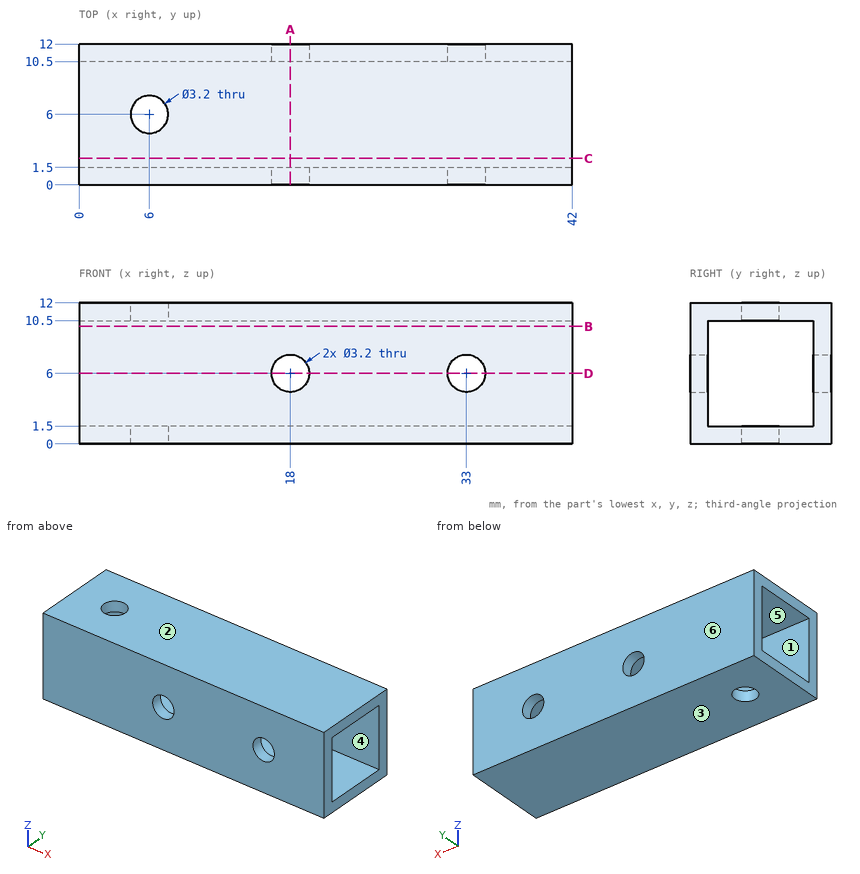
Can you work these out from the drawing? Everything is in mm from the part's minimum corner. A direction names the side the tool comes from. Coordinates: 2 decimals unless noted, no trailing zeros. Loops run counter-clockwise (first coordinate to the right, second up) from the corner with the lowest first, then second, coordinate; pieces in that order, holes last. Notation, with made-up numbers: (78.5, 22.25) - (102.5, 22.25) arc R18 cw to (102.5, 52.25) - close; hole circle Ø10 at (79, 40). An arc over 180 degrees is marked (long way). Use a Markdown table: item, result.
Item 1: I want a section at B-B on z = 10. Please give me the cut outline in (x, y).
Numbers:
| item | result |
|---|---|
| outline | (0, 0) - (42, 0) - (42, 1.5) - (0, 1.5) - close; (0, 10.5) - (42, 10.5) - (42, 12) - (0, 12) - close |
Item 2: For the marked faces 5 and 6, which set-ups out of +Z, -Z, +X, -X, +Y, -Y let a thin tool reach every point of the face, with its end or its side?
Numbers:
| item | result |
|---|---|
| face 5 | +X, -X |
| face 6 | +Z, -Z, +X, -X, +Y |
Item 3: We'd pull the mould along Z, two halves only. Please class the marked faces 1, 2, 3 and 4: released by +Z, released by -Z, zero draft, split by the parting line, or undercut.
Numbers:
| item | result |
|---|---|
| face 1 | undercut |
| face 2 | released by +Z |
| face 3 | released by -Z |
| face 4 | undercut |
Item 4: I want a section at D-D on z = 6. Please give me the cut outline in (x, y).
Numbers:
| item | result |
|---|---|
| outline | (0, 0) - (16.4, 0) - (16.4, 1.5) - (0, 1.5) - close; (0, 10.5) - (16.4, 10.5) - (16.4, 12) - (0, 12) - close; (19.6, 0) - (31.4, 0) - (31.4, 1.5) - (19.6, 1.5) - close; (19.6, 10.5) - (31.4, 10.5) - (31.4, 12) - (19.6, 12) - close; (34.6, 0) - (42, 0) - (42, 1.5) - (34.6, 1.5) - close; (34.6, 10.5) - (42, 10.5) - (42, 12) - (34.6, 12) - close |
Item 5: I want a section at A-A on x = 18. Please give me the cut outline in (y, z), and give its area (3 significant figures).
Numbers:
| item | result |
|---|---|
| outline | (0, 0) - (12, 0) - (12, 4.4) - (10.5, 4.4) - (10.5, 1.5) - (1.5, 1.5) - (1.5, 4.4) - (0, 4.4) - close; (0, 7.6) - (1.5, 7.6) - (1.5, 10.5) - (10.5, 10.5) - (10.5, 7.6) - (12, 7.6) - (12, 12) - (0, 12) - close |
| area | 53.4 mm2 |
Item 6: If I drill on probe 1 along X at (y, z) = (10.8, 6); probe 2 along Y at (x, z) = (27, 6.5); probe 3 along Z at (x, y) = (18, 11.6), over which ranges is the centre line in solid material (lowest first)? Write a range as from..to.
Numbers:
| item | result |
|---|---|
| probe 1 | x = 0..16.4, 19.6..31.4, 34.6..42 |
| probe 2 | y = 0..1.5, 10.5..12 |
| probe 3 | z = 0..4.4, 7.6..12 |
